Part model, mm, in its own coordinate system. Face numbers are marked on the shaded views. A direction names the side the tool comes from. Give positions to 0.01 mm unless a question says otherwise; leave off trailing zeros. Order: outer loops, then holes, each group sorted by start corner. A loop starts at its lowest first (then second) coordinate and runs counter-clockwise, first axis right, second up. Notation, with made-up numbers: (-34, 37.25) -> (14, 37.25) arc R18 cw to (14, 42.25) -> close; hole circle Ø3 at (53.5, 70.25). An arc over 180 degrees is marked (long way). Write item = value, one per line. Start each with the question number.
(1) Saw through at D-D, the plane y = 42.5. List the corners of the cut face in (x, z), then the cut area to 3 significant figures.
(2) Which spindle directions (+Z, -Z, +X, -X, +Y, -Y) get a long thin tool onto all of the face, cutting with end or side? Do the marked faces 1, 2 and 3. Say none if no direction does.
(3) Saw through at C-C, the plane z = -46. List the corners of the cut face in (x, y), then the cut area to 3 significant figures.
(4) Probe line 1 along X through (y, z) = (10, -49.35); line 2 along Y through (x, z) = (15, -15); line 3 along Y through (x, z) = (29.5, -43.5). List the from-to ranges inside material, lowest first. Write a range as from..to.
(5) Saw through at A-A, the plane y = 60. List the corners of the cut face in (x, z).
(6) Two-plate mould, pull along Y, no slides. Class the marked faces 4, 5, 6 and 7: pulls with the +Y half, pulls with the -Y half, needs draft (parallel to the pull), parting line crosses it, or undercut.
(7) Saw through at B-B, the plane x = 8. List the corners of the cut face in (y, z) (3 decimals), then the cut area to 3 significant figures.
(8) Flat gauge pins, fed straight in: pin 1 (6.5 mm diameter, centred on x = 45, y = 10, fed in from +Z); pin 2 (12 mm diameter, centred on y = 61.5, z = -19, fed in from -X); pin 3 (2 mm diameter, centred on x = 35.5, y = 36.5, fed in from +Z) (3 decimals); pin 4 (22 mm diameter, centred on x = 45, y = 5.5, fed in from -Z) (3 decimals). Where does each tip first touch, or does it go through?
from build123d import *

# Parameters (mm, degrees)
BOSS_EXTRUDE1_DEPTH = 60
SKETCH3_R           = 5.05
CUT_EXTRUDE1_DEPTH  = 70
SKETCH4_R           = 13.05
CUT_EXTRUDE2_DEPTH  = 8
SKETCH5_R           = 2.5
CUT_EXTRUDE3_DEPTH  = 61
SKETCH6_R           = 5
CUT_EXTRUDE4_DEPTH  = 12
SKETCH7_W           = 20
SKETCH7_H           = 50
CUT_EXTRUDE5_DEPTH  = 81


with BuildPart() as part:
    # Sketch2 → Boss-Extrude1 (new body)
    with BuildSketch(Plane(origin=(0, 0, 0), x_dir=(0, 0, -1), z_dir=(1, 0, 0))):
        Polygon((0, 40), (10, 0), (19.925, 0), (19.925, 20), (40.075, 20), (40.075, 0), (50, 0), (60, 40), (60, 80), (50, 120), (40.075, 120), (40.075, 100), (19.925, 100), (19.925, 120), (10, 120), (0, 80), align=None)
    extrude(amount=BOSS_EXTRUDE1_DEPTH)

    # Sketch3 → Cut-Extrude1 (cut)
    with BuildSketch(Plane.XY):
        with Locations((30, 60)):
            Circle(SKETCH3_R)
    extrude(amount=-CUT_EXTRUDE1_DEPTH, mode=Mode.SUBTRACT)

    # Sketch4 → Cut-Extrude2 (cut)
    with BuildSketch(Plane.XY):
        with Locations((30, 60)):
            Circle(SKETCH4_R)
    cut_extrude2 = extrude(amount=-CUT_EXTRUDE2_DEPTH, mode=Mode.SUBTRACT)

    # Mirror1: Cut-Extrude2 across plane
    add(cut_extrude2.mirror(Plane.XY.offset(-30)), mode=Mode.SUBTRACT)

    # Sketch5 → Cut-Extrude3 (cut, through all)
    with BuildSketch(Plane.XY):
        with Locations((45, 110)):
            Circle(SKETCH5_R)
        with Locations((15, 110)):
            Circle(SKETCH5_R)
        with Locations((45, 10)):
            Circle(SKETCH5_R)
        with Locations((15, 10)):
            Circle(SKETCH5_R)
    extrude(amount=-CUT_EXTRUDE3_DEPTH, mode=Mode.SUBTRACT)

    # Sketch6 → Cut-Extrude4 (cut)
    with BuildSketch(Plane.XY):
        with Locations((45, 110)):
            Circle(SKETCH6_R)
        with Locations((15, 110)):
            Circle(SKETCH6_R)
        with Locations((15, 10)):
            Circle(SKETCH6_R)
        with Locations((45, 10)):
            Circle(SKETCH6_R)
    cut_extrude4 = extrude(amount=-CUT_EXTRUDE4_DEPTH, mode=Mode.SUBTRACT)

    # Mirror2: Cut-Extrude4 across plane
    add(cut_extrude4.mirror(Plane.XY.offset(-30)), mode=Mode.SUBTRACT)

    # Sketch7 → Cut-Extrude5 (cut)
    with BuildSketch(Plane(origin=(60, 0, 0), x_dir=(0, 0, -1), z_dir=(1, 0, 0))):
        with Locations((30, 60)):
            Rectangle(SKETCH7_W, SKETCH7_H)
    extrude(amount=-CUT_EXTRUDE5_DEPTH, mode=Mode.SUBTRACT)


solid = part.part
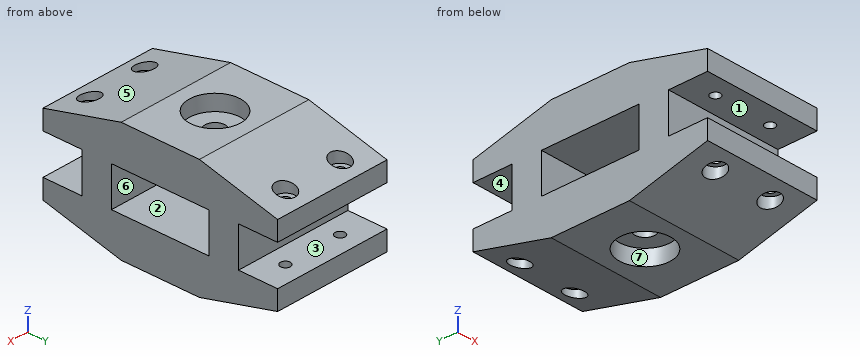
Results list:
q1.outline = (0, -60) -> (60, -60) -> (60, -40) -> (0, -40) -> close; (0, -20) -> (60, -20) -> (60, 0) -> (0, 0) -> close
q1.area = 2,400 mm^2
q2.face_1 = +X, -X, -Y
q2.face_2 = +X, -X
q2.face_3 = +X, -X, +Y
q3.outline = (0, 0) -> (60, 0) -> (60, 120) -> (0, 120) -> close; hole circle Ø5 at (15, 10); hole circle Ø5 at (15, 110); hole circle Ø10.1 at (30, 60); hole circle Ø5 at (45, 10); hole circle Ø5 at (45, 110)
q3.area = 7,040 mm^2
q4.line_1 = 0..10, 20..40, 50..60
q4.line_2 = 0..7.5, 12.5..107.5, 112.5..120
q4.line_3 = 0..54.97, 65.03..120
q5.outline = (0, -60) -> (16.95, -60) -> (16.95, -52) -> (24.95, -52) -> (24.95, -40) -> (0, -40) -> close; (0, -20) -> (24.95, -20) -> (24.95, -8) -> (16.95, -8) -> (16.95, 0) -> (0, 0) -> close; (35.05, -52) -> (43.05, -52) -> (43.05, -60) -> (60, -60) -> (60, -40) -> (35.05, -40) -> close; (35.05, -20) -> (60, -20) -> (60, 0) -> (43.05, 0) -> (43.05, -8) -> (35.05, -8) -> close
q6.face_4 = needs draft
q6.face_5 = pulls with the -Y half
q6.face_6 = undercut
q6.face_7 = undercut
q7.outline = (0, -50) -> (40, -60) -> (80, -60) -> (120, -50) -> (120, -40.075) -> (100, -40.075) -> (100, -19.925) -> (120, -19.925) -> (120, -10) -> (80, 0) -> (40, 0) -> (0, -10) -> (0, -19.925) -> (20, -19.925) -> (20, -40.075) -> (0, -40.075) -> close; hole (35, -40) -> (85, -40) -> (85, -20) -> (35, -20) -> close
q7.area = 4,590 mm^2
q8.pin_1 = -12
q8.pin_2 = 0
q8.pin_3 = -0.625
q8.pin_4 = -54.125
